Check sheet for the modelled part. Datum: model origin and axes. Units: mm. A direction names the side the tool comes from. Round coordinates to 2 decimals unless told otherwise and drop trailing zeros. Write each loop counter-clockwise with the first axis right and the second up, starting at its lowest first coordinate (ties: lowest second). Pieces come first, ordered by that corner, then holes.
Item 1: Material ranges on line 1 (Y direction, x = 18.2, z = -29.8); line 2 (Y direction, x = -6.5, z = 6.5); line 3 (Z direction, x = 18.75, y = 18.75), recorded low to high.
Item 2: Cross-section at A-A on z = 6.5. Enter the section's corners in (x, y), plus the area to 3 significant figures.
Item 3: Cross-section at C-C on x = 15.5. Enter the section's corners in (y, z).
Item 4: Cross-section at D-D on z = -15. Enter the section's corners in (x, y) (3 decimals).
Item 5: Cross-section at B-B on y = 16. Enter the section's corners in (x, z), plus the area to 3 significant figures.
Item 6: Release check for a two-part mould opening along Z. For faces 1 (the flat face through (13.97, 12, -16)), 2 (the cylindrical face through (17.012, 20.425, -2.644)), 3 (the flat face through (17, 18, -27.854)), 4 (the cylindrical face through (-5.972, 12.859, 10.797)) record: +Z half, -Z half, draft (parallel to the pull), parting line (faces both ways), or undercut.
Item 7: Go/stop test with flat-tipped pins: pin 1 Ø4 at (x, z) = (-2.5, -15.5) entering from +Y; pin 2 Ø6 at (x, y) = (9, 10) entering from -Z; pin 3 Ø5 at (x, z) = (5, -24.5) entering from +Y. Record where each tip stops, or that it passes through.
Item 8: Tool access check on faces 5 (the flat face through (17, 12.954, -16)), 6 (the cylindrical face through (16.93, 24.53, -28.42)), 7 (the flat face through (0, 12, -17)), 8 (the flat face through (3.897, 7.611, -16.072)), 9 (the flat face through (10.5, 6.6, -32.6)). Record the directions out of +Z, -Z, +X, -X, +Y, -Y that give a thin tool (end or side, any length) a straight path to the whole face; none if there is none.
Autodesk Inventor part; units mm, degrees
ref_plane "YZ Plane" through (0, 0, 0) normal (1, 0, 0) x (0, 1, 0)
ref_plane "XZ Plane" through (0, 0, 0) normal (0, 1, 0) x (-1, 0, 0)
ref_plane "XY Plane" through (0, 0, 0) normal (0, 0, 1) x (1, 0, 0)
sketch "Náčrt1" plane through (0, 0, 0) normal (0, 0, 1) x (1, 0, 0)
  line L0 (13.97, 23.865) -> (13.97, 9.144)
  line L1 (0, 9.144) -> (0, 0)
  line L2 (4.5409, 9.144) -> (0, 9.144)
  line L3 (4.5409, 8.255) -> (4.5409, 9.144)
  line L4 (3.2709, 6.985) -> (4.5409, 8.255)
  line L5 (3.2709, 4.318) -> (3.2709, 6.985)
  line L6 (8.7319, 9.144) -> (8.7319, 8.255)
  line L7 (13.97, 9.144) -> (8.7319, 9.144)
  line L8 (8.7319, 8.255) -> (10.0019, 6.985)
  line L9 (10.0019, 6.985) -> (10.0019, 4.318)
  line L10 (10.0019, 4.318) -> (3.2709, 4.318)
  line L11 (0, 0) -> (19.97, 0)
  line L12 (13.97, 22.5956) -> (13.97, 25.1349)
  line L13 (13.97, 20.4353) -> (13.97, 18.035)
  line L14 (13.97, 25.1349) -> (19.97, 25.1349)
  line L15 (19.97, 25.1349) -> (19.97, 0)
extrude "Vysunutí1" add sketch "Náčrt1" against normal blind 32.6
sketch "Náčrt2" plane through (19.97, 0, 0) normal (1, 0, 0) x (0, 0, -1)
  line L0 (0, 25.1349) -> (32.6, 25.1349)
  line L1 (16.3, 25.1349) -> (4.746, 25.1349)
  line L2 (4.746, 25.1349) -> (4.746, 12.9539)
  line L3 (16.3, 25.1349) -> (27.854, 25.1349)
  line L4 (27.854, 25.1349) -> (27.854, 12.9539)
  line L5 (27.854, 12.9539) -> (4.746, 12.9539)
  circle A0 centre (2.8, 19.2349) radius 1.2
  line L6 (16.3, 25.1349) -> (16.3, 15.9225)
  circle A1 centre (29.8, 19.2349) radius 1.2
  point P0 (0, 0)
  point P1 (4.746, 19.0444)
  dimension "d2" = 11.554
  dimension "d3" = 12.181
  dimension "d4" = 11.554
  dimension "d7" = 2.4
  dimension "d8" = 5.9
  dimension "d9" = 1.946
extrude "Vysunutí2" cut sketch "Náčrt2" against normal blind 32.6 contours L0 L4 L5 L2
extrude "Vysunutí3" cut sketch "Náčrt2" against normal blind 32.6 contours A0 | A1
fillet "Zaoblení1" radius 2 4 edges at (16.97, 25.1349, 0) (16.97, 25.1349, -4.746) (16.97, 25.1349, -27.854) (16.97, 25.1349, -32.6)
sketch "Náčrt3" plane through (0, 0, 0) normal (0, -1, 0) x (1, 0, 0)
  point P0 (0, 0)
sketch "Náčrt4" plane through (0, 0, 0) normal (0, 0, 1) x (1, 0, 0)
  line L0 (13.97, 23.1349) -> (19.97, 23.1349)
  line L1 (13.97, 23.1349) -> (13.97, 9.144)
  line L2 (13.97, 9.144) -> (8.7319, 9.144)
  line L3 (8.7319, 9.144) -> (8.7319, 8.255)
  line L4 (8.7319, 8.255) -> (10.0019, 6.985)
  line L5 (10.0019, 6.985) -> (10.0019, 4.318)
  line L6 (10.0019, 4.318) -> (3.2709, 4.318)
  line L7 (3.2709, 4.318) -> (3.2709, 6.985)
  line L8 (3.2709, 6.985) -> (4.5409, 8.255)
  line L9 (4.5409, 8.255) -> (4.5409, 9.144)
  line L10 (4.5409, 9.144) -> (0, 9.144)
  line L11 (0, 9.144) -> (0, 0)
  line L12 (0, 0) -> (19.97, 0)
  line L13 (19.97, 0) -> (19.97, 23.1349)
  line L14 (0, 0) -> (-8, 0)
  line L15 (-8, 0) -> (-8, 14)
  line L16 (-8, 14) -> (0, 14)
  line L17 (0, 14) -> (0, 0)
  dimension "d13" = 14
  dimension "d14" = 8
extrude "Vysunutí4" add sketch "Náčrt4" along normal blind 12 and the other way blind 32.6 contours L14 L15 L16 L17 L11
sketch "Náčrt5" plane through (0, 0, 0) normal (1, 0, 0) x (0, 0, -1)
  line L0 (0, 9.144) -> (0, 0)
  line L1 (0, 9.144) -> (32.6, 9.144)
  line L2 (32.6, 14) -> (32.6, 9.144)
  line L3 (32.6, 14) -> (-12, 14)
  line L4 (-12, 0) -> (-12, 14)
  line L5 (0, 0) -> (-12, 0)
  circle A0 centre (-6.5, 7) radius 2.25
  line L6 (27.854, 12.9539) -> (4.746, 12.9539)
  line L7 (16.3, 12.9539) -> (16.3, -5.3216)
  line L8 (32.6, 9.144) -> (32.6, 0)
  line L9 (44.6, 0) -> (44.6, 14)
  line L10 (32.6, 0) -> (44.6, 0)
  circle A1 centre (39.1, 7) radius 2.25
  line L11 (44.6, 14) -> (32.6, 14)
  line L12 (32.6, 14) -> (32.6, 0)
  dimension "d19" = 4.5
  dimension "d20" = 7
  dimension "d21" = 5.5
extrude "Vysunutí5" add sketch "Náčrt5" against normal up to surface (8 mm away) contours L2 L11 L9 L10 L8 | A0
sketch "Náčrt6" plane through (0, 0, 12) normal (0, 0, 1) x (1, 0, 0)
  line L0 (-8, 14) -> (-8, 0)
  line L1 (-8, 0) -> (0, 0)
  line L2 (0, 0) -> (0, 14)
  line L3 (0, 14) -> (-8, 14)
  line L4 (0, 14) -> (-4, 14)
  line L5 (-4, 14) -> (-4, 0)
  line L6 (-4, 0) -> (0, 0)
  line L7 (0, 0) -> (0, 14)
  dimension "d24" = 4
extrude "Vysunutí6" cut sketch "Náčrt6" against normal blind 12 contours L3 L2 L1 L5
extrude "Vysunutí7" cut sketch "Náčrt5" against normal blind 4 contours L2 L11 L9 L10 L8 | A0
sketch "Náčrt7" plane through (-4, 0, 12) normal (1, 0, 0) x (0, 0, -1)
  circle A0 centre (51.1, 7) radius 2.25
  line L0 (0, 0) -> (0, 14)
  line L1 (12, 0) -> (0, 0)
  line L2 (12, 0) -> (12, 14)
  line L3 (0, 14) -> (12, 14)
  line L4 (44.6, 0) -> (44.6, 14)
  line L5 (56.6, 0) -> (44.6, 0)
  line L6 (56.6, 14) -> (56.6, 0)
  line L7 (44.6, 14) -> (56.6, 14)
  circle A1 centre (51.1, 7) radius 2.25
  line L8 (12, 0) -> (44.6, 0)
  circle A2 centre (5.5, 7) radius 2.25
  line L9 (44.6, 14) -> (12, 14)
  point P0 (0, 7)
  dimension "d29" = 4.5
  dimension "d30" = 5.5
extrude "Vysunutí8" cut sketch "Náčrt7" against normal blind 4 contours A2
fillet "Zaoblení2" radius 4 4 edges at (-6, 14, -44.6) (-6, 0, -44.6) (-6, 14, 12) (-6, 0, 12)
properties part number "Motor_holder_Vertical" material "Měď"
Response values:
1. line 1: y = 0 to 18.03, 20.43 to 25.13
1. line 2: y = 0 to 4.75, 9.25 to 14
1. line 3: z = -32.6 to -30.9, -28.7 to -27.85, -4.75 to -3.9, -1.7 to 0
2. outline: (-8, 0) - (-4, 0) - (-4, 4.75) - (-8, 4.75) - close; (-8, 9.25) - (-4, 9.25) - (-4, 14) - (-8, 14) - close
2. area: 38.0 mm2
3. outline: (0, -32.6) - (23.13, -32.6) arc R2 ccw to (25.13, -30.6) - (25.13, -29.85) arc R2 ccw to (23.13, -27.85) - (12.95, -27.85) - (12.95, -4.75) - (23.13, -4.75) arc R2 ccw to (25.13, -2.75) - (25.13, -2) arc R2 ccw to (23.13, 0) - (0, 0) - close; hole circle Ø2.4 at (19.23, -29.8); hole circle Ø2.4 at (19.23, -2.8)
4. outline: (-8, 0) - (19.97, 0) - (19.97, 12.954) - (13.97, 12.954) - (13.97, 9.144) - (8.732, 9.144) - (8.732, 8.255) - (10.002, 6.985) - (10.002, 4.318) - (3.271, 4.318) - (3.271, 6.985) - (4.541, 8.255) - (4.541, 9.144) - (0, 9.144) - (0, 14) - (-8, 14) - close
5. outline: (13.97, -32.6) - (19.97, -32.6) - (19.97, -27.85) - (13.97, -27.85) - close; (13.97, -4.75) - (19.97, -4.75) - (19.97, 0) - (13.97, 0) - close
5. area: 57.0 mm2
6. face 1: draft
6. face 2: undercut
6. face 3: undercut
6. face 4: +Z half
7. pin 1: stops at y = 14
7. pin 2: stops at z = -32.6
7. pin 3: stops at y = 9.14
8. face 5: +X, +Y
8. face 6: +X, -X, +Y
8. face 7: +Z, -Z, +Y
8. face 8: +Z, -Z
8. face 9: -Z, +X, +Y, -Y
